Part model, mm, in its own coordinate system. Face numbers are marked on the shaded views. A direction names the side the tool comes from. Give positions to 0.01 mm unless a question says otherwise; leave off trailing zeros. Order: outer loops, then holes, each group sorted by start corner. A loop starts at its lowest first (then second) coordinate and runs counter-clockwise, first axis right, second up. Notation, with made-up numbers: M -23,70 L -10,70 A29 cw -10,105 Z; hole C 89.5,34 d2. An arc over 180 degrees is marked long. One line per question, with ' | ' between items.
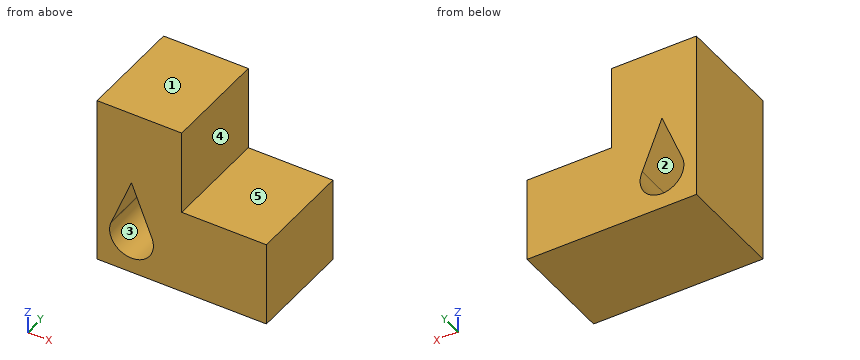
```python
from build123d import *

# Parameters (mm, degrees)
F0_W     = 20
F0_H     = 20
F1_DEPTH = 25


with BuildPart() as f1:
    # F0 (on Front) → F1 (new body)
    with BuildSketch(Plane.XZ):
        Polygon((0, 4.873418), (0, 0), (20, 0), (20, 20), (20, 40), (0, 40), align=None)
        with BuildLine():
            ThreePointArc((3.263231, 10.481385), (3.330913, 10.659271), (3.405091, 10.834548))
            Line((3.405091, 10.834548), (8.132556, 22.603722))
            Line((8.132556, 22.603722), (12.795818, 10.973252))
            ThreePointArc((12.795818, 10.973252), (8.399199, 3.562881), (3.263231, 10.481385))
        make_face(mode=Mode.SUBTRACT)
        with Locations((30, 10)):
            Rectangle(F0_W, F0_H)
    extrude(amount=F1_DEPTH)


solid = f1.part
```
1. Slice it at B-B on z = 15. Give the cut face in (x, y).
Worked out:
outline: M 0,-25 L 5.08,-25 L 5.08,0 L 0,0 Z; M 11.18,-25 L 40,-25 L 40,0 L 11.18,0 Z
2. Slice it at D-D on z = 28. Give the cut face in (x, y).
Worked out:
outline: M 0,-25 L 20,-25 L 20,0 L 0,0 Z
3. Drop flat-ended pins along their axis: pin 1 (8 mm diameter, centred on y = -10, z = 25.5, fed in from +X); pin 2 (6 mm diameter, centred on x = 33, y = -6.5, fed in from +Z). Give the stop position or say it passes through.
Worked out:
pin 1: stops at x = 20 | pin 2: stops at z = 20
4. Slice it at A-A on y = -18.25. Give the cut face in (x, z).
Worked out:
outline: M 0,0 L 40,0 L 40,20 L 20,20 L 20,40 L 0,40 Z; hole M 3.26,10.48 A5.17 ccw long 12.8,10.97 L 8.13,22.6 L 3.41,10.83 A5.17 ccw Z
5. Slice it at C-C on x = 9. Give the cut face in (y, z).
Worked out:
outline: M -25,0 L 0,0 L 0,3.63 L -25,3.63 Z; M -25,20.44 L 0,20.44 L 0,40 L -25,40 Z
6. Probe L1, parallel to Z at x = 38.5, y = -6.25; L2, parallel to X at y = -7.5, z = 18.5. List the from-to ranges inside material, lowest first. Write a range as from..to.
Worked out:
L1: z = 0..20 | L2: x = 0..6.48, 9.78..40
7. Mould opens along X. For the marked faces 3, 4 and 5 say: released by +X, released by -X, zero draft, split by the parting line, or undercut.
Worked out:
face 3: undercut | face 4: released by +X | face 5: zero draft
8. Tool access for the marked faces 1 and 2: list every direction of +Z, -Z, +X, -X, +Y, -Y with a clear straight run to the whole face (end or side of a thin tool).
Worked out:
face 1: +Z, +X, -X, +Y, -Y | face 2: +Y, -Y
